Build history of the part. All positions in model axes, mm. Face numbers are marked on the shaded views. A direction names the side the tool comes from. Give positions to 0.01 mm unless a question says otherwise; leave off trailing zeros. Write each loop counter-clockwise with the first axis right and the second up, starting at its lowest first coordinate (ties: lowest second). Pieces come first, ordered by that corner, then holes. Notation, with made-up numbers: (-3.75, 74.5) -> (20.25, 74.5) arc R11 ccw to (20.25, 89.5) -> close; hole circle Ø4 at (57.5, -6). An arc over 180 degrees is marked (long way). Put each result on its own line as item: value. Start each with the question number.
Item 1: Slice it at C-C, the plane y = -1.75. List the corners of the cut face in (x, z).
Item 2: Flat gauge pins, fed straight in: pin 1 Ø3 at (x, z) = (11.5, -3.5) entering from -Y; pin 2 Ø5 at (x, z) = (10.5, -0.5) entering from -Y; pin 3 Ø2.5 at (y, z) = (-4, 0) entering from +X; pin 4 Ø0.6 at (x, z) = (18.5, 5) entering from +Y. Where does each tip first touch, or does it go through?
Item 3: Slice it at D-D, the plane x = 15.5. List the corners of the cut face in (y, z), plus the area to 3 significant figures.
Item 4: Drill centre lines: line 1 along X through (y, z) = (-5, 0.25); line 2 along Y through (x, z) = (10.75, 0); line 3 along Y through (x, z) = (18.85, 0). Where is each one in solid material? Low to high.
Item 5: Slice it at A-A, the plane z = 6.5. List the corners of the cut face in (x, y).
Item 6: Two-plate mould, pull along X, no slides. Class the marked faces 4, 5 and 6: pulls with the +X half, pulls with the -X half, needs draft (parallel to the pull), parting line crosses it, or undercut.
Item 7: Slice it at B-B, the plane z = 0. List the corners of the cut face in (x, y), plus the area to 3 significant figures.
Item 8: Tool access for the marked faces 1, 2 and 3: list every direction of +Z, -Z, +X, -X, +Y, -Y with a clear straight run to the whole face (end or side of a thin tool).
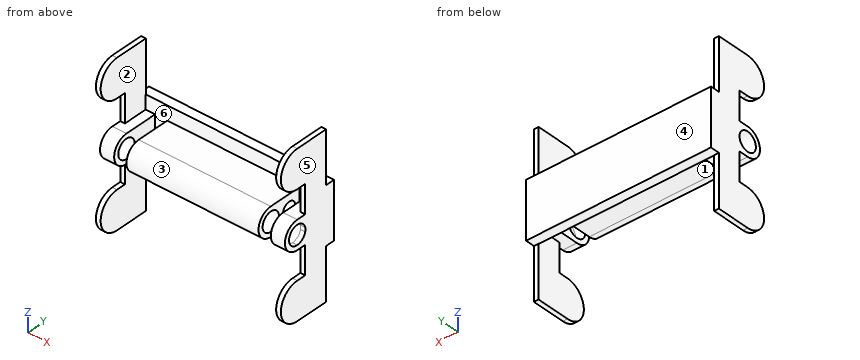
```python
from build123d import *

# Parameters (mm, degrees)
SKETCH1_R           = 1.001
SKETCH1_W           = 6
SKETCH1_H           = 1
BOSS_EXTRUDE1_DEPTH = 18.604
CUT_EXTRUDE1_REACH  = 8
SKETCH2_W           = 1.302
SKETCH2_H           = 5.804323037
SKETCH2_H_2         = 5.909581117
CUT_EXTRUDE2_REACH  = 18.302
SKETCH3_R           = 0.75
BOSS_EXTRUDE2_DEPTH = 0.5


with BuildPart() as part:
    # Sketch1 → Boss-Extrude1 (new body)
    with BuildSketch(Plane(origin=(0, 0, 0), x_dir=(0, 0, -1), z_dir=(1, 0, 0))):
        with BuildLine():
            Line((1.5, -4), (1.5, -0.5))
            Line((1.5, -0.5), (-1.5, -0.5))
            Line((-1.5, -0.5), (-1.5, -4))
            ThreePointArc((-1.5, -4), (0, -5.5), (1.5, -4))
        make_face()
        with Locations((0, -4)):
            Circle(SKETCH1_R, mode=Mode.SUBTRACT)
        Rectangle(SKETCH1_W, SKETCH1_H)
    extrude(amount=BOSS_EXTRUDE1_DEPTH)

    # Sketch2 → Cut-Extrude1 (cut, up to next)
    with BuildSketch(Plane.XY.offset(3), mode=Mode.PRIVATE) as cut_extrude1_sk1:
        with Locations((1.651, -3.402161519)):
            Rectangle(SKETCH2_W, SKETCH2_H)
    cut_extrude1_tool1 = extrude(cut_extrude1_sk1.sketch, amount=-CUT_EXTRUDE1_REACH, mode=Mode.PRIVATE) & part.part
    add(cut_extrude1_tool1.solids().sort_by_distance((1.651, -3.402162, 3))[0], mode=Mode.SUBTRACT)
    # Sketch2 → Cut-Extrude1 (cut, up to next)
    with BuildSketch(Plane.XY.offset(3), mode=Mode.PRIVATE) as cut_extrude1_sk2:
        with Locations((16.953, -3.454790559)):
            Rectangle(SKETCH2_W, SKETCH2_H_2)
    cut_extrude1_tool2 = extrude(cut_extrude1_sk2.sketch, amount=-CUT_EXTRUDE1_REACH, mode=Mode.PRIVATE) & part.part
    add(cut_extrude1_tool2.solids().sort_by_distance((16.953, -3.454791, 3))[0], mode=Mode.SUBTRACT)

    # Sketch3 → Cut-Extrude2 (cut, up to next)
    with BuildSketch(Plane.ZY.offset(-2.302), mode=Mode.PRIVATE) as cut_extrude2_sk1:
        with Locations((0, -1.75)):
            Circle(SKETCH3_R)
    cut_extrude2_tool1 = extrude(cut_extrude2_sk1.sketch, amount=-CUT_EXTRUDE2_REACH, mode=Mode.PRIVATE) & part.part
    add(cut_extrude2_tool1.solids().sort_by_distance((2.302, -1.75, 0))[0], mode=Mode.SUBTRACT)

    # Sketch4 → Boss-Extrude2 (add)
    with BuildSketch(Plane(origin=(18.604, 0, 0), x_dir=(0, 0, -1), z_dir=(1, 0, 0))):
        with BuildLine():
            Line((-4.5, -4), (-4.5, -3.026257348))
            Line((-4.5, -3.026257348), (-1.5, -3.026257348))
            Line((-1.5, -3.026257348), (-1.5, -4))
            ThreePointArc((-1.5, -4), (0, -5.5), (1.5, -4))
            Line((1.5, -4), (1.5, -3.026257348))
            Line((1.5, -3.026257348), (4.5, -3.026257348))
            Line((4.5, -3.026257348), (4.5, -4))
            ThreePointArc((4.5, -4), (6.5, -6), (8.5, -4))
            Line((8.5, -4), (8.5, -3.026257348))
            Line((8.5, -3.026257348), (8.5, -0.472742652))
            Line((8.5, -0.472742652), (3, -0.472742652))
            Line((3, -0.472742652), (3, 0.5))
            Line((3, 0.5), (-3, 0.5))
            Line((-3, 0.5), (-3, -0.472742652))
            Line((-3, -0.472742652), (-8.5, -0.472742652))
            Line((-8.5, -0.472742652), (-8.5, -3.026257348))
            Line((-8.5, -3.026257348), (-8.5, -4))
            ThreePointArc((-8.5, -4), (-6.5, -6), (-4.5, -4))
        make_face()
        with BuildLine():
            ThreePointArc((1.001, -4), (-0.620388649, -4.785569173), (-0.232004845, -3.026257348))
            ThreePointArc((-0.232004845, -3.026257348), (0, -2.999), (0.232004845, -3.026257348))
            ThreePointArc((0.232004845, -3.026257348), (0.785569173, -3.379611351), (1.001, -4))
        make_face(mode=Mode.SUBTRACT)
    boss_extrude2 = extrude(amount=BOSS_EXTRUDE2_DEPTH)

    # Mirror2: Boss-Extrude2 across plane
    add(boss_extrude2.mirror(Plane.ZY.offset(-9.302)))


solid = part.part
```
Values follow:
1. outline: (-0.5, -8.5) -> (0, -8.5) -> (0, -1.5) -> (1, -1.5) -> (1, 1.5) -> (0, 1.5) -> (0, 8.5) -> (-0.5, 8.5) -> close; (2.3, -1.5) -> (16.3, -1.5) -> (16.3, -0.75) -> (2.3, -0.75) -> close; (2.3, 0.75) -> (16.3, 0.75) -> (16.3, 1.5) -> (2.3, 1.5) -> close; (17.6, -1.5) -> (18.6, -1.5) -> (18.6, -8.5) -> (19.1, -8.5) -> (19.1, 8.5) -> (18.6, 8.5) -> (18.6, 1.5) -> (17.6, 1.5) -> close
2. pin 1: y = -0.5
2. pin 2: y = -5.5
2. pin 3: x = 19.1
2. pin 4: y = -0.47
3. outline: (-4, -1.5) -> (-0.5, -1.5) -> (-0.5, -3) -> (0.5, -3) -> (0.5, 3) -> (-0.5, 3) -> (-0.5, 1.5) -> (-4, 1.5) arc R1.5 ccw to start; hole circle Ø2 at (-4, 0); hole circle Ø1.5 at (-1.75, 0)
3. area: 15.1 mm2
4. line 1: -0.5 to 1, 2.3 to 16.3, 17.6 to 19.1
4. line 2: -5.5 to -5, -3 to -2.5, -1 to 0.5
4. line 3: -5.5 to -5, -3 to 0.5
5. outline: (-0.5, -6) -> (0, -6) -> (0, -0.47) -> (-0.5, -0.47) -> close; (18.6, -6) -> (19.1, -6) -> (19.1, -0.47) -> (18.6, -0.47) -> close
6. face 4: needs draft
6. face 5: pulls with the +X half
6. face 6: undercut
7. outline: (-0.5, -5.5) -> (1, -5.5) -> (1, -5) -> (-0.5, -5) -> close; (-0.5, -3) -> (1, -3) -> (1, -0.5) -> (2.3, -0.5) -> (2.3, -1) -> (16.3, -1) -> (16.3, -0.5) -> (17.6, -0.5) -> (17.6, -3) -> (19.1, -3) -> (19.1, 0.5) -> (-0.5, 0.5) -> close; (2.3, -5.5) -> (16.3, -5.5) -> (16.3, -5) -> (2.3, -5) -> close; (2.3, -3) -> (16.3, -3) -> (16.3, -2.5) -> (2.3, -2.5) -> close; (17.6, -5.5) -> (19.1, -5.5) -> (19.1, -5) -> (17.6, -5) -> close
7. area: 49.6 mm2
8. face 1: -Z, -Y
8. face 2: +Z, -Y
8. face 3: +X, -X, -Y
